Model file for the job. Use its own axes, mm. A direction names the side the tool comes from. Round coordinates to 2 decimals unless told otherwise and drop trailing zeros. Order: outer loops, then holes, each group sorted by start corner. A loop starts at its lowest first (then second) coordinate and runs counter-clockwise, first axis right, second up. Notation, with made-up numbers: (69, 57.25) - (86, 57.25) arc R9 ccw to (86, 74.25) - close; hole circle Ø3 at (26.5, -2). An arc over 180 degrees is marked (long way). Write item = value, one per line.
```python
from build123d import *

# Parameters (mm, degrees)
SKETCH1_R           = 2.032
BOSS_EXTRUDE1_DEPTH = 19.05
BOSS_EXTRUDE2_START = 3.175
BOSS_EXTRUDE2_DEPTH = 3.175
FILLET1_R           = 1.27
SKETCH3_R           = 1.905
CUT_EXTRUDE1_DEPTH  = 52.21483461447027


with BuildPart() as part:
    # Sketch1 → Boss-Extrude1 (new, symmetric)
    # profile 1 of 2: a face of its own
    with BuildSketch(Plane.XY):
        with BuildLine():
            Line((0, 50.8), (0, 25.40000000000009))
            Line((0, 25.40000000000009), (4.803171045006462, 20.59682895499363))
            ThreePointArc((4.803171045006465, 20.59682895499363), (7.897944154578656, 39.95075151177493), (21.589999999999996, 53.97499999999999))
            Line((21.589999999999996, 53.974999999999994), (21.589999999999996, 63.5))
            Line((21.589999999999996, 63.5), (0, 63.5))
            Line((0, 63.5), (0, 50.8))
        make_face()
        with Locations(Location((6.35, 44.449999999999996, 0), (0, 0, 180))):
            Circle(SKETCH1_R, mode=Mode.SUBTRACT)
    # profile 2 of 2: a face of its own
    with BuildSketch(Plane.XY):
        with BuildLine():
            Line((0, 50.8), (0, 25.40000000000009))
            Line((0, 25.40000000000009), (4.803171045006462, 20.59682895499363))
            ThreePointArc((4.803171045006465, 20.59682895499363), (7.897944154578656, 39.95075151177493), (21.589999999999996, 53.97499999999999))
            Line((21.589999999999996, 53.974999999999994), (21.589999999999996, 63.5))
            Line((21.589999999999996, 63.5), (0, 63.5))
            Line((0, 63.5), (0, 50.8))
        make_face()
        with Locations(Location((6.35, 44.449999999999996, 0), (0, 0, 180))):
            Circle(SKETCH1_R, mode=Mode.SUBTRACT)
    extrude(amount=BOSS_EXTRUDE1_DEPTH, both=True)

    # Sketch2 → Boss-Extrude2 (add)
    with BuildSketch(Plane.XY.offset(19.05).offset(BOSS_EXTRUDE2_START)):
        with BuildLine():
            Line((0, 63.5), (21.589999999999996, 63.5))
            Line((21.589999999999996, 63.5), (21.589999999999996, 53.974999999999994))
            ThreePointArc((21.589999999999996, 53.974999999999994), (19.09356210818939, 52.4962542782198), (16.7394991351634, 50.8))
            Line((16.7394991351634, 50.8), (1.56e-15, 50.8))
            Line((1.56e-15, 50.8), (0, 63.5))
        make_face()
    boss_extrude2 = extrude(amount=-BOSS_EXTRUDE2_DEPTH)

    # Mirror1: Boss-Extrude2 across plane
    add(boss_extrude2.mirror(Plane.XY))

    # Fillet1
    fillet1_edges = [part.edges().sort_by_distance(p)[0] for p in [
        (4.803171045006463, 20.59682895499363, 0),
        (0, 25.40000000000009, 0),
        (0, 63.5, 0),
        (21.589999999999996, 63.5, 0),
        (21.589999999999996, 53.974999999999994, 0),
        (1.56e-15, 50.8, 20.637500000000003),
        (16.7394991351634, 50.8, 20.637500000000003),
        (1.56e-15, 50.8, -20.637500000000003),
        (16.7394991351634, 50.8, -20.637500000000003),
    ]]
    fillet(fillet1_edges, radius=FILLET1_R)

    # Sketch3 → Cut-Extrude1 (cut, through all)
    with BuildSketch(Plane(origin=(0, 63.5, 0), x_dir=(1, 0, 0), z_dir=(0, 1, 0))):
        with Locations(Location((13.335, -11.430000000000003, 0), (0, 0, 270))):
            Circle(SKETCH3_R)
    extrude(amount=-CUT_EXTRUDE1_DEPTH, mode=Mode.SUBTRACT)


solid = part.part
```
1) Cut at C-C (x = 5.25). Write the cut outline in (y, z) (3 decimals), and give its area (3 significant figures).
Conclusion:
outline = (32.576, -19.05) - (42.741, -19.05) - (42.741, 19.05) - (32.576, 19.05) - close; (46.159, -19.05) - (50.8, -19.05) - (50.8, -22.225) - (63.5, -22.225) - (63.5, 22.225) - (50.8, 22.225) - (50.8, 19.05) - (46.159, 19.05) - close
area = 1,130 mm^2
2) 3-axis set-ups, long thin cutter, end or side, ignore diameter. For faces 4 (the face through (11, 57, 22.225)), 5 (the face through (9, 50.8, 21)), 6 (the face through (0.382, 51.162, -20.615)): which of +Z, -Z, +X, -X, +Y, -Y reach the whole face in a straight line?
Conclusion:
face_4 = +Z, +X, -X, +Y, -Y
face_5 = +Z, +X, -X, -Y
face_6 = -Z, -X, -Y
3) Cut at D-D (z = -2.5). Write the cut outline in (x, y) (3 decimals).
Conclusion:
outline = (0, 25.926) arc R1.27 ccw to (0.372, 25.028) - (2.306, 23.094) arc R1.27 ccw to (4.473, 24.045) arc R32.385 cw to (20.943, 53.62) arc R1.27 ccw to (21.59, 54.727) - (21.59, 62.23) arc R1.27 ccw to (20.32, 63.5) - (1.27, 63.5) arc R1.27 ccw to (0, 62.23) - close; hole circle Ø4.064 at (6.35, 44.45)
4) Flat gauge pins, fed straight in: pin 1 Ø1.6 at (x, z) = (8.5, -21) entering from -Y; pin 2 Ø4 at (x, y) = (8, 33.5) entering from -Z; pin 3 Ø5 at (y, z) = (42.5, 11) entering from +X; pin 4 Ø5.5 at (x, y) = (6.35, 44.45) entering from -Z. Where does each tip first touch, or does it go through?
Conclusion:
pin_1 = 50.8
pin_2 = through
pin_3 = 11.05
pin_4 = -19.05
5) Mould opens along X. For faces 1 (the face through (0.382, 51.162, 20.615)), 2 (the face through (9, 50.8, -21)), 3 (the face through (11.475, 54.621, 11.017)) say: +X half, -X half, draft (parallel to the pull), parting line (faces both ways), or undercut.
Conclusion:
face_1 = -X half
face_2 = draft
face_3 = undercut
6) Wall check: line 1 along X through (y, z) = (60, 11.43); line 2 along Z through (x, y) = (4, 27); line 3 along X through (y, z) = (44, 2). Give the ranges that are in metal, low to high.
Conclusion:
line_1 = 0 to 11.43, 15.24 to 21.59
line_2 = -19.05 to 19.05
line_3 = 0 to 4.37, 8.33 to 10.32
7) Cut at B-B (y = 44.45). Write the cut outline in (x, z), and give its area (3 significant figures).
Conclusion:
outline = (0, -19.05) - (4.32, -19.05) - (4.32, 19.05) - (0, 19.05) - close; (8.38, -19.05) - (10.64, -19.05) - (10.64, 19.05) - (8.38, 19.05) - close
area = 251 mm^2
8) Cut at A-A (z = 11.43). Give the number of separate pieces and of enclosed holes in the cut face, and give its area (3 significant figures).
Conclusion:
separate_pieces = 2
enclosed_holes = 1
area = 407 mm^2
